```python
from build123d import *

# Parameters (mm, degrees)
F1_DEPTH = 26
F2_R     = 5
F3_DEPTH = 36.001
F4_R     = 5


with BuildPart() as f1:
    # F0 (on Top) → F1 (new body)
    with BuildSketch(Plane.XY):
        Polygon((-16, 15), (-18, 15), (-18, -15), (18, -15), (18, 15), (16, 15), (16, -13), (-16, -13), align=None)
    extrude(amount=F1_DEPTH)

    # F2 (on face) → F3 (cut, through all)
    with BuildSketch(Plane.YZ.offset(18)):
        with Locations((0, 13)):
            Circle(F2_R)
    extrude(amount=-F3_DEPTH, mode=Mode.SUBTRACT)

    # F4
    f4_edges = [f1.edges().sort_by_distance(p)[0] for p in [
        (17, 15, 0),
        (-17, 15, 0),
        (-17, 15, 26),
        (17, 15, 26),
    ]]
    fillet(f4_edges, radius=F4_R)


solid = f1.part
```
Source: CAD feature listing. Evaluate the final solid. Frame: model axes, mm. A direction names the side the tool comes from. Give positions to 0.01 mm unless a question says otherwise; leave off trailing zeros. Write each loop counter-clockwise with the first axis right and the second up, starting at its lowest first coordinate (ties: lowest second). Pieces come first, ordered by that corner, then holes.
1. Access query for faces 4 (the face through (0, -15, 13)), 5 (the face through (0, -13, 13)). Directions: +Z, -Z, +X, -X, +Y, -Y. A direction counts if a zero-diameter tool reaches every point of the face in a straight line with its end or side. Return the directions, or none.
2. Section query B-B (z = 13). Return the cut outline in (x, y), then the cut area to 3 significant figures.
3. Section query D-D (z = 24). Return the cut outline in (x, y).
4. Section query A-A (y = 4). Return the cut outline in (x, z), then the cut area to 3 significant figures.
5. Pull-direction query (Z, two-part tool) for faces 1 (the face through (17, 13, 25)), 2 (the face through (-16.986, -0.651, 17.957)), 3 (the face through (-18, 0, 19)); classes: +Z half, -Z half, draft (parallel to the pull), parting line (faces both ways), or undercut.
6. First-contact query: pin 1 (1.5 mm diameter, centred on x = -13, z = 19.5, fed in from +Y). Flat tip, straight axial feed; report the tip coordinate or a pass-through.
7. Section query C-C (y = -7.25). Return the cut outline in (x, z), then the cut area to 3 significant figures.
8. Material intervals for line 1 along Z through (x, y) = (-16.35, 0); line 2 along X through (y, z) = (11.25, 9); line 3 along Y through (x, z) = (-7, 11.5), sorted ascending.
Output values:
1. face 4: +Z, -Z, +X, -X, -Y
1. face 5: +Z, -Z, +Y
2. outline: (-18, -15) - (18, -15) - (18, -5) - (16, -5) - (16, -13) - (-16, -13) - (-16, -5) - (-18, -5) - close; (-18, 5) - (-16, 5) - (-16, 15) - (-18, 15) - close; (16, 5) - (18, 5) - (18, 15) - (16, 15) - close
2. area: 144 mm2
3. outline: (-18, -15) - (18, -15) - (18, 14) - (16, 14) - (16, -13) - (-16, -13) - (-16, 14) - (-18, 14) - close
4. outline: (-18, 0) - (-16, 0) - (-16, 10) - (-18, 10) - close; (-18, 16) - (-16, 16) - (-16, 26) - (-18, 26) - close; (16, 0) - (18, 0) - (18, 10) - (16, 10) - close; (16, 16) - (18, 16) - (18, 26) - (16, 26) - close
4. area: 80.0 mm2
5. face 1: +Z half
5. face 2: undercut
5. face 3: draft
6. pin 1: stops at y = -13
7. outline: (-18, 0) - (-16, 0) - (-16, 26) - (-18, 26) - close; (16, 0) - (18, 0) - (18, 26) - (16, 26) - close
7. area: 104 mm2
8. line 1: z = 0 to 8, 18 to 26
8. line 2: x = -18 to -16, 16 to 18
8. line 3: y = -15 to -13
